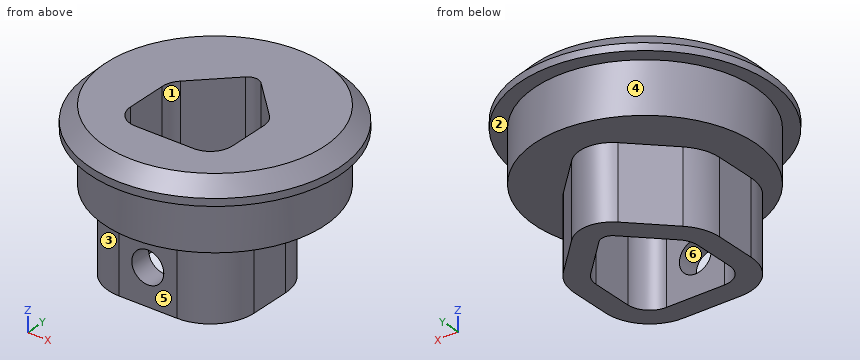
from build123d import *

# Parameters (mm, degrees)
F3_DEPTH = 10.001
F5_DEPTH = 10
F6_R     = 2.2
F7_DEPTH = 3


with BuildPart() as f1:
    # F0 (on Right) → F1 (revolve)
    with BuildSketch(Plane.YZ):
        Polygon((-15, 0), (0, 0), (0, 10), (-15, 10), (-17, 8), (-17, 7), (-15, 7), align=None)
    revolve(axis=Axis((0, 0, -2.15537), (0, 0, -1)))

    # F2 (on face) → F3 (cut, through all)
    with BuildSketch(Plane.XY.offset(10)):
        with BuildLine():
            Line((-7, -0.343146), (-7, -6))
            ThreePointArc((-7, -6), (-6.12132, -8.12132), (-4, -9))
            Line((-4, -9), (4, -9))
            ThreePointArc((4, -9), (6.12132, -8.12132), (7, -6))
            Line((7, -6), (7, -0.343146))
            ThreePointArc((7, -0.343146), (6.771639, 0.804905), (6.12132, 1.778175))
            Line((6.12132, 1.778175), (1.06066, 6.838835))
            ThreePointArc((1.06066, 6.838835), (0, 7.278175), (-1.06066, 6.838835))
            Line((-1.06066, 6.838835), (-6.12132, 1.778175))
            ThreePointArc((-6.12132, 1.778175), (-6.771639, 0.804905), (-7, -0.343146))
        make_face()
    extrude(amount=-F3_DEPTH, mode=Mode.SUBTRACT)

    # F4 (on face) → F5 (join)
    with BuildSketch(Plane(origin=(0, 0, 0), x_dir=(1, 0, 0), z_dir=(0, 0, -1))):
        with BuildLine():
            Line((4, 12), (-4, 12))
            ThreePointArc((-4, 12), (-8.242641, 10.242641), (-10, 6))
            Line((-10, 6), (-10, 0.343146))
            ThreePointArc((-10, 0.343146), (-9.543277, -1.952955), (-8.242641, -3.899495))
            Line((-8.242641, -3.899495), (-3.181981, -8.960155))
            ThreePointArc((-3.181981, -8.960155), (0, -10.278175), (3.181981, -8.960155))
            Line((3.181981, -8.960155), (8.242641, -3.899495))
            ThreePointArc((8.242641, -3.899495), (9.543277, -1.952955), (10, 0.343146))
            Line((10, 0.343146), (10, 6))
            ThreePointArc((10, 6), (8.242641, 10.242641), (4, 12))
        make_face()
        with BuildLine():
            ThreePointArc((-7, 6), (-6.12132, 8.12132), (-4, 9))
            Line((-4, 9), (4, 9))
            ThreePointArc((4, 9), (6.12132, 8.12132), (7, 6))
            Line((7, 6), (7, 0.343146))
            ThreePointArc((7, 0.343146), (6.771639, -0.804905), (6.12132, -1.778175))
            Line((6.12132, -1.778175), (1.06066, -6.838835))
            ThreePointArc((1.06066, -6.838835), (0, -7.278175), (-1.06066, -6.838835))
            Line((-1.06066, -6.838835), (-6.12132, -1.778175))
            ThreePointArc((-6.12132, -1.778175), (-6.771639, -0.804905), (-7, 0.343146))
            Line((-7, 0.343146), (-7, 6))
        make_face(mode=Mode.SUBTRACT)
    extrude(amount=F5_DEPTH)

    # F6 (on face) → F7 (cut, through all)
    with BuildSketch(Plane.XZ.offset(12)):
        with Locations((0, -5)):
            Circle(F6_R)
    extrude(amount=-F7_DEPTH, mode=Mode.SUBTRACT)


solid = f1.part
Geometry: final body of the model. Coordinates: model frame, mm. Face numbers are marked on the shaded views. A direction names the side the tool comes from. Give positions to 0.01 mm unless a question says otherwise; leave off trailing zeros. Loops run counter-clockwise (first coordinate to the right, second up) from the corner with the lowest first, then second, coordinate; pieces in that order, holes last. Notation, with made-up numbers: (1, 59) - (11, 59) arc R13 cw to (11, 72) - close; hole circle Ø8 at (-6, 29.5). An arc over 180 degrees is marked (long way). Answer as CSV lines item,"result". Start each with the question number.
1. Section D-D, the plane z = -8.5. Return loops of the section in (x, y).
2. Section C-C, the plane z = -5. Return loops of the section in (x, y), plus the area to 3 significant figures.
3. Pin query (flat end, axial travel): P1, Ø2, axis at x = 2, z = -3.5, coming from the -Y side; P2, Ø12, axis at y = 12, z = 4.5, coming from the +X side; P3, Ø3.5, axis at x = 0, z = -5, coming from the -Y side; P4, Ø8, axis at x = -12.5, y = 4, coming from the -Z side. Return the tip coordinate at first contact, or that it passes through.
4. Section A-A, the plane z = 1.5. Return loops of the section in (x, y), plus the area to 3 significant figures.
5. Ray query, L1, parallel to Z at x = 0, y = -10; L2, parallel to X at y = -2, z = -3.5; L3, parallel to X at y = -7, z = -8. Return the intervals inside material, ascending.
6. Reachability of the marked faces 4, 5 and 6 from +Z, -Z, +X, -X, +Y, -Y: full face, straight path, thin tool, end or side. Return the list, or none.
7. Section B-B, the plane x = 0. Return loops of the section in (y, z), plus the area to 3 significant figures.
8. Draft query along X for the marked faces 1, 2 and 3. Return one class per face: released by +X, released by -X, zero draft, split by the parting line, or undercut.
Answers:
1,outline,"(-10, -6) arc R6 ccw to (-4, -12) - (4, -12) arc R6 ccw to (10, -6) - (10, -0.34) arc R6 ccw to (8.24, 3.9) - (3.18, 8.96) arc R4.5 ccw to (-3.18, 8.96) - (-8.24, 3.9) arc R6 ccw to (-10, -0.34) - close; hole (-7, -6) arc R3 ccw to (-4, -9) - (4, -9) arc R3 ccw to (7, -6) - (7, -0.34) arc R3 ccw to (6.12, 1.78) - (1.06, 6.84) arc R1.5 ccw to (-1.06, 6.84) - (-6.12, 1.78) arc R3 ccw to (-7, -0.34) - close"
2,outline,"(-10, -6) arc R6 ccw to (-4, -12) - (-2.2, -12) - (-2.2, -9) - (-4, -9) arc R3 cw to (-7, -6) - (-7, -0.34) arc R3 cw to (-6.12, 1.78) - (-1.06, 6.84) arc R1.5 cw to (1.06, 6.84) - (6.12, 1.78) arc R3 cw to (7, -0.34) - (7, -6) arc R3 cw to (4, -9) - (2.2, -9) - (2.2, -12) - (4, -12) arc R6 ccw to (10, -6) - (10, -0.34) arc R6 ccw to (8.24, 3.9) - (3.18, 8.96) arc R4.5 ccw to (-3.18, 8.96) - (-8.24, 3.9) arc R6 ccw to (-10, -0.34) - close"
2,area,"165 mm2"
3,P1,"stops at y = -12"
3,P2,"stops at x = 15.69"
3,P3,"stops at y = 6.15"
3,P4,"stops at z = -10"
4,outline,"circle Ø30 at (0, 0); hole (-7, -6) arc R3 ccw to (-4, -9) - (4, -9) arc R3 ccw to (7, -6) - (7, -0.34) arc R3 ccw to (6.12, 1.78) - (1.06, 6.84) arc R1.5 ccw to (-1.06, 6.84) - (-6.12, 1.78) arc R3 ccw to (-7, -0.34) - close"
4,area,"524 mm2"
5,L1,"z = -10 to -7.2, -2.8 to 10"
5,L2,"x = -10 to -7, 7 to 10"
5,L3,"x = -9.92 to -6.83, 6.83 to 9.92"
6,face 4,"-Z"
6,face 5,"-Z, +X, -X, -Y"
6,face 6,"-Y"
7,outline,"(-17, 7) - (-15, 7) - (-15, 0) - (-12, 0) - (-12, -2.8) - (-9, -2.8) - (-9, 10) - (-15, 10) - (-17, 8) - close; (-12, -10) - (-9, -10) - (-9, -7.2) - (-12, -7.2) - close; (7.28, -10) - (10.28, -10) - (10.28, 0) - (15, 0) - (15, 7) - (17, 7) - (17, 8) - (15, 10) - (7.28, 10) - close"
7,area,"192 mm2"
8,face 1,"undercut"
8,face 2,"zero draft"
8,face 3,"released by -X"
